```python
from build123d import *

# Parameters (mm, degrees)
SKETCH1_R           = 20
BOSS_EXTRUDE1_DEPTH = 12.7
SKETCH2_R           = 1.5875
CUT_EXTRUDE1_DEPTH  = 89.674827911
SKETCH3_W           = 21.981677087
SKETCH3_H           = 54.692506085
SKETCH3_W_2         = 54.954192717
SKETCH3_H_2         = 20.019027347
CUT_EXTRUDE2_DEPTH  = 70.866
SKETCH4_R           = 3.175
CUT_EXTRUDE3_DEPTH  = 13.462
SKETCH5_R           = 3.175
CUT_EXTRUDE4_DEPTH  = 13.462


with BuildPart() as part:
    # Sketch1 → Boss-Extrude1 (new body)
    with BuildSketch(Plane(origin=(0, 0, 0), x_dir=(0, 0, -1), z_dir=(1, 0, 0))):
        with BuildLine():
            Line((0, 34.177299494), (34.177299494, 34.177299494))
            Line((34.177299494, 34.177299494), (63.133299494, 34.177299494))
            Line((63.133299494, 34.177299494), (63.133299494, -60.96))
            Line((63.133299494, -60.96), (-34.177299494, -60.96))
            Line((-34.177299494, -60.96), (-34.177299494, 0))
            ThreePointArc((-34.177299494, 0), (-24.167000235, 24.167000235), (0, 34.177299494))
        make_face()
        Circle(SKETCH1_R, mode=Mode.SUBTRACT)
    extrude(amount=BOSS_EXTRUDE1_DEPTH)

    # Sketch2 → Cut-Extrude1 (cut, through all)
    with BuildSketch(Plane(origin=(0, 0, 0), x_dir=(1, 0, 0), z_dir=(0, 1, 0))):
        with Locations(Location((6.35, 0, 0), (0, 0, 90))):
            Circle(SKETCH2_R)
    extrude(amount=CUT_EXTRUDE1_DEPTH, mode=Mode.SUBTRACT)

    # Sketch3 → Cut-Extrude2 (cut)
    with BuildSketch(Plane.ZY):
        with Locations((-45.095335943, 0.281776268)):
            Rectangle(SKETCH3_W, SKETCH3_H)
        with Locations((1.22319792, -44.53205946)):
            Rectangle(SKETCH3_W_2, SKETCH3_H_2)
        with Locations((-45.095335943, -44.53205946)):
            Rectangle(SKETCH3_W, SKETCH3_H_2)
    extrude(amount=-CUT_EXTRUDE2_DEPTH, mode=Mode.SUBTRACT)

    # Sketch4 → Cut-Extrude3 (cut)
    with BuildSketch(Plane.XZ.offset(60.96)):
        with Locations(Location((6.35, 16.646444295, 0), (0, 0, 270))):
            Circle(SKETCH4_R)
        with Locations(Location((6.35, -45.192507654, 0), (0, 0, 270))):
            Circle(SKETCH4_R)
    extrude(amount=-CUT_EXTRUDE3_DEPTH, mode=Mode.SUBTRACT)

    # Sketch5 → Cut-Extrude4 (cut)
    with BuildSketch(Plane(origin=(0, 0, -63.133299494), x_dir=(-1, 0, 0), z_dir=(0, 0, -1))):
        with Locations((-6.35, 17.445139987)):
            Circle(SKETCH5_R)
        with Locations((-6.35, -44.233190942)):
            Circle(SKETCH5_R)
    extrude(amount=-CUT_EXTRUDE4_DEPTH, mode=Mode.SUBTRACT)


solid = part.part
```
Verification items for the finished model (mm, model axes). A direction names the side the tool comes from. Coordinates: 2 decimals unless noted, no trailing zeros. Loops run counter-clockwise (first coordinate to the right, second up) from the corner with the lowest first, then second, coordinate; pieces in that order, holes last. Notation, with made-up numbers: (-38.75, -29) - (-7.75, -29) arc R30 cw to (-7.75, 6) - close; hole circle Ø7 at (13, 47.25). An arc over 180 degrees is marked (long way). Answer as a JSON object with one key per item and string values.
(1) Scan lines: line 1 along Z through (x, y) = (2, -0.5); line 2 along Z through (x, y) = (6.5, -56); line 3 along Z through (x, y) = (6.25, -26.5). Record each from-to range of solid material in increasing order.
Response:
{"line 1": "z = -63.13 to -56.09, -34.1 to -19.99, 19.99 to 34.18", "line 2": "z = -63.13 to -48.36, -42.02 to 13.47, 19.82 to 34.18", "line 3": "z = -63.13 to -56.09, -34.1 to 34.18"}
(2) Cross-section at B-B, the plane y = -1.5. Record the boundary of the cut face in (x, z), then the cut area to 3 significant figures.
Response:
{"outline": "(0, -63.13) - (12.7, -63.13) - (12.7, -56.09) - (0, -56.09) - close; (0, -34.1) - (12.7, -34.1) - (12.7, -19.94) - (0, -19.94) - close; (0, 19.94) - (12.7, 19.94) - (12.7, 34.18) - (0, 34.18) - close", "area": "450 mm²"}
(3) Cross-section at D-D, the plane z = -4. Record the boundary of the cut face in (x, y), then the cut area to 3 significant figures.
Response:
{"outline": "(0, -60.96) - (12.7, -60.96) - (12.7, -54.54) - (0, -54.54) - close; (0, -34.52) - (12.7, -34.52) - (12.7, -19.6) - (0, -19.6) - close; (0, 19.6) - (12.7, 19.6) - (12.7, 34.18) - (0, 34.18) - close", "area": "456 mm²"}
(4) Mould release check, pull along X, two halves, no side actions. Record for faces 1 (the flat face through (9, -42, -56.086)), 2 (the cylindrical face through (8.496, -57.796, -42.852)), 3 (the cylindrical face through (7.038, -47.333, -59.659)), 4 (the flat face through (12.7, -23, -15)): pulls with the +X half, pulls with the -X half, needs draft (parallel to the pull), parting line crosses it, or undercut.
Response:
{"face 1": "needs draft", "face 2": "undercut", "face 3": "undercut", "face 4": "pulls with the +X half"}
(5) Access from +Z, -Z, +X, -X, +Y, -Y to the whole of each face (thin tool, end or side, straight path). Record for faces 5 (the flat face through (6, -13, -63.133)), 6 (the flat face through (6, -27.064, -45)), 7 (the cylindrical face through (8.496, -57.796, 18.987)), 8 (the cylindrical face through (7.038, 14.346, -59.659)).
Response:
{"face 5": "-Z, +X, -X, +Y, -Y", "face 6": "+X, -X", "face 7": "-Y", "face 8": "-Z"}
(6) Cross-section at C-C, the plane x = 10.75. Record the boundary of the cut face in (y, z), then the cut area to 3 significant figures.
Response:
{"outline": "(-60.96, -63.13) - (34.18, -63.13) - (34.18, 0) arc R34.18 ccw to (0, 34.18) - (-60.96, 34.18) - close; hole (-54.54, -56.09) - (-34.52, -56.09) - (-34.52, -34.1) - (-54.54, -34.1) - close; hole (-54.54, -26.25) - (-34.52, -26.25) - (-34.52, 28.7) - (-54.54, 28.7) - close; hole (-27.06, -56.09) - (27.63, -56.09) - (27.63, -34.1) - (-27.06, -34.1) - close; hole circle Ø40 at (0, 0)", "area": "5,010 mm²"}
(7) Go/stop test with flat-tipped pins: pin 1 Ø6.5 at (x, z) = (6, -45) entering from -Y; pin 2 Ø8 at (y, z) = (-15.5, -3) entering from +X. Record where each tip stops, or that it passes through.
Response:
{"pin 1": "stops at y = -60.96", "pin 2": "passes through"}
(8) Cross-section at A-A, the plane z = -22. Record the boundary of the cut face in (x, y).
Response:
{"outline": "(0, -60.96) - (12.7, -60.96) - (12.7, -54.54) - (0, -54.54) - close; (0, -34.52) - (12.7, -34.52) - (12.7, 34.18) - (0, 34.18) - close"}
